Drawing for the job (mm, zero at the part's lowest x, y, z). A direction names the side the tool comes from. Round coordinates to 2 decimals unless told otherwise and drop trailing zeros. Write each loop counter-clockwise with the first axis right and the second up, starting at its lowest first coordinate (ties: lowest second). Pieces come first, ordered by that corner, then holes.
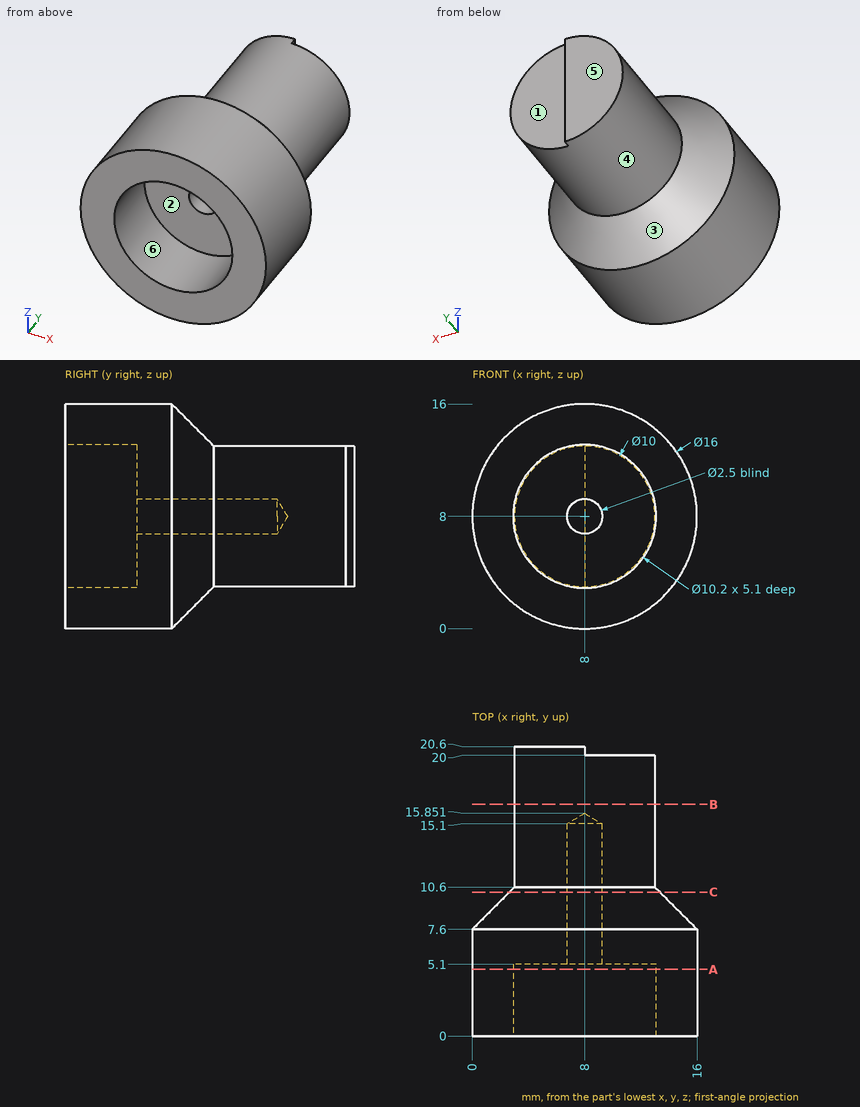
Q1. Saw through at A-A, the plane y = 4.75. Write the cut outline in (x, z), and give its area (3 significant figures).
Q2. Tool access for the marked faces 4, 5 and 6: list every direction of +Z, -Z, +X, -X, +Y, -Y with a clear straight run to the whole face (end or side of a thin tool).
Q3. Wall check: line 1 (Z direction, x = 8, y = 2.75); line 2 (Z direction, x = 8, y = 10.5); line 3 (Y direction, x = 9, z = 3.25). Give the ranges that are in metal, low to high.
Q4. Saw through at C-C, the plane y = 10.25. Write the cut outline in (x, z), and give its area (3 significant figures).
Q5. Two-plate mould, pull along Z, no slides. Class the marked faces 1, 2 and 3: released by +Z, released by -Z, zero draft, split by the parting line, or undercut.
Q6. Drop flat-ended pins along their axis: P1, Ø5, axis at x = 8, z = 9.5, coming from the -Y side; P2, Ø1, axis at y = 7.5, z = 10, coming from the +X side; P3, Ø3, axis at x = 10, z = 6, coming from the +Y side. Give the stop position or say it passes through.
Q7. Saw through at B-B, the plane y = 16.5. Write the cut outline in (x, z).
Computed:
1. outline: circle Ø16 at (8, 8); hole circle Ø10.2 at (8, 8)
1. area: 119 mm2
2. face 4: +Y
2. face 5: +Z, -Z, +X, -X, +Y
2. face 6: -Y
3. line 1: z = 0 to 2.9, 13.1 to 16
3. line 2: z = 2.9 to 6.75, 9.25 to 13.1
3. line 3: y = 5.1 to 20
4. outline: circle Ø10.7 at (8, 8); hole circle Ø2.5 at (8, 8)
4. area: 85.0 mm2
5. face 1: zero draft
5. face 2: undercut
5. face 3: split by the parting line
6. P1: stops at y = 5.1
6. P2: stops at x = 15.86
6. P3: stops at y = 20
7. outline: circle Ø10 at (8, 8)
